The model under review builds one solid part; all positions refer to its coordinate system, in mm. A direction names the side the tool comes from. Round coordinates to 2 decimals unless told otherwise and drop trailing zeros. Write each loop counter-clockwise with the first axis right and the second up, starting at its lowest first coordinate (ties: lowest second). Pieces come first, ordered by that corner, then holes.
Item 1: Clearance check with flat-ended pins moving along their axes: pin 1 Ø2.5 at (x, z) = (27.5, -2.5) entering from +Y; pin 2 Ø1.5 at (y, z) = (173.5, -2.5) entering from -X; pin 3 Ø1.5 at (x, z) = (23, -3) entering from +Y. State where each tip first meets the part, or that it passes through.
Item 2: Draft analysis for pull direction Y (two halves, no side actions). For faces 6 (the face through (40, 190.358, -2)), 7 (the face through (25, 73, -2)), 8 (the face through (47.5, -2, -2)), state which applies: +Y half, -Y half, draft (parallel to the pull), parting line (faces both ways), or undercut.
Item 3: Add section A-A (x = 22.5). Give the boundary of the cut face in (y, z), plus the area to 3 significant figures.
Item 4: Machinability: for faces 1 (the face through (52.5, 91, -2)), 2 (the face through (23, 102.5, -2)), 3 (the face through (22, 42.5, -2)), 4 (the face through (25, 164, -2)), 5 (the face through (50, 185.358, -2)), which of the approach directions +Z, -Z, +X, -X, +Y, -Y give a long, thin tool a straight path to every point of the face, cutting with its end or side? Answer none if there is none.
Item 5: Add section B-B (z = -1.35). Give the boundary of the cut face in (x, y), plus the area to 3 significant figures.
Item 6: To check wall thickness, follow L1, parallel to Y at x = 22.5, z = -4.55; L2, parallel to X at y = 179, z = -4.1; L3, parallel to Y at x = 30, z = -3.7. State the ranges of each line that lie inside material, in increasing order.
Item 7: Add section C-C (y = 173). Give the boundary of the cut face in (x, z), plus the area to 4 significant figures.
```python
from build123d import *

# Parameters (mm, degrees)
BOSS_EXTRUDE1_DEPTH = 5


with BuildPart() as part:
    # Sketch1 → Boss-Extrude1 (new body)
    with BuildSketch(Plane.XY):
        Polygon((52.5, 185.35845109), (47.5, 185.35845109), (47.5, 190.35845109), (32.5, 190.35845109), (32.5, 185.35845109), (25, 185.35845109), (25, 142.5), (20, 142.5), (20, 122.5), (25, 122.5), (25, 102.5), (20, 102.5), (20, 82.5), (25, 82.5), (25, 62.5), (20, 62.5), (20, 42.5), (25, 42.5), (25, 0), (32.5, 0), (32.5, -4.64154891), (40, -4.64154891), (47.5, -4.64154891), (47.5, 0), (52.5, 0), align=None)
    extrude(amount=-BOSS_EXTRUDE1_DEPTH)


solid = part.part
```
Numbers:
1. pin 1: stops at y = 185.36
1. pin 2: stops at x = 25
1. pin 3: stops at y = 142.5
2. face 6: +Y half
2. face 7: undercut
2. face 8: draft
3. outline: (42.5, -5) - (62.5, -5) - (62.5, 0) - (42.5, 0) - close; (82.5, -5) - (102.5, -5) - (102.5, 0) - (82.5, 0) - close; (122.5, -5) - (142.5, -5) - (142.5, 0) - (122.5, 0) - close
3. area: 300 mm2
4. face 1: +Z, -Z, +X, +Y, -Y
4. face 2: +Z, -Z, -X
4. face 3: +Z, -Z, -X, -Y
4. face 4: +Z, -Z, -X, +Y
4. face 5: +Z, -Z, +X, +Y
5. outline: (20, 42.5) - (25, 42.5) - (25, 0) - (32.5, 0) - (32.5, -4.64) - (47.5, -4.64) - (47.5, 0) - (52.5, 0) - (52.5, 185.36) - (47.5, 185.36) - (47.5, 190.36) - (32.5, 190.36) - (32.5, 185.36) - (25, 185.36) - (25, 142.5) - (20, 142.5) - (20, 122.5) - (25, 122.5) - (25, 102.5) - (20, 102.5) - (20, 82.5) - (25, 82.5) - (25, 62.5) - (20, 62.5) - close
5. area: 5,540 mm2
6. L1: y = 42.5 to 62.5, 82.5 to 102.5, 122.5 to 142.5
6. L2: x = 25 to 52.5
6. L3: y = 0 to 185.36
7. outline: (25, -5) - (52.5, -5) - (52.5, 0) - (25, 0) - close
7. area: 137.5 mm2
